Part print with two shaded views. Sizes in mm from the minimum x, y, z corner. A direction names the side the tool comes from. Coordinates: 2 decimals unless noted, no trailing zeros. Return JSON: item names as keys, results as strings. Group by question number.
(1) Flat gauge pins, fed straight in: pin 1 Ø12 at (x, z) = (252, 97) entering from -Y (3 decimals); pin 2 Ø3 at (x, y) = (267.5, 3.5) entering from +Z. Where does each tip first touch, or does it go through?
(2) Tool access for the marked faces 5 and 6: list every direction of +Z, -Z, +X, -X, +Y, -Y with a clear straight run to the whole face (end or side of a thin tool).
(3) Mould opens along Y. For the marked faces 1, 2, 3 and 4 say: pulls with the +Y half, pulls with the -Y half, needs draft (parallel to the pull), parting line crosses it, or undercut.
(4) Probe L1, parallel to Y at x = 463, z = 78 (1 decimal); L2, parallel to Z at x = 66.5, y = 49.5. List the from-to ranges inside material, lowest first.
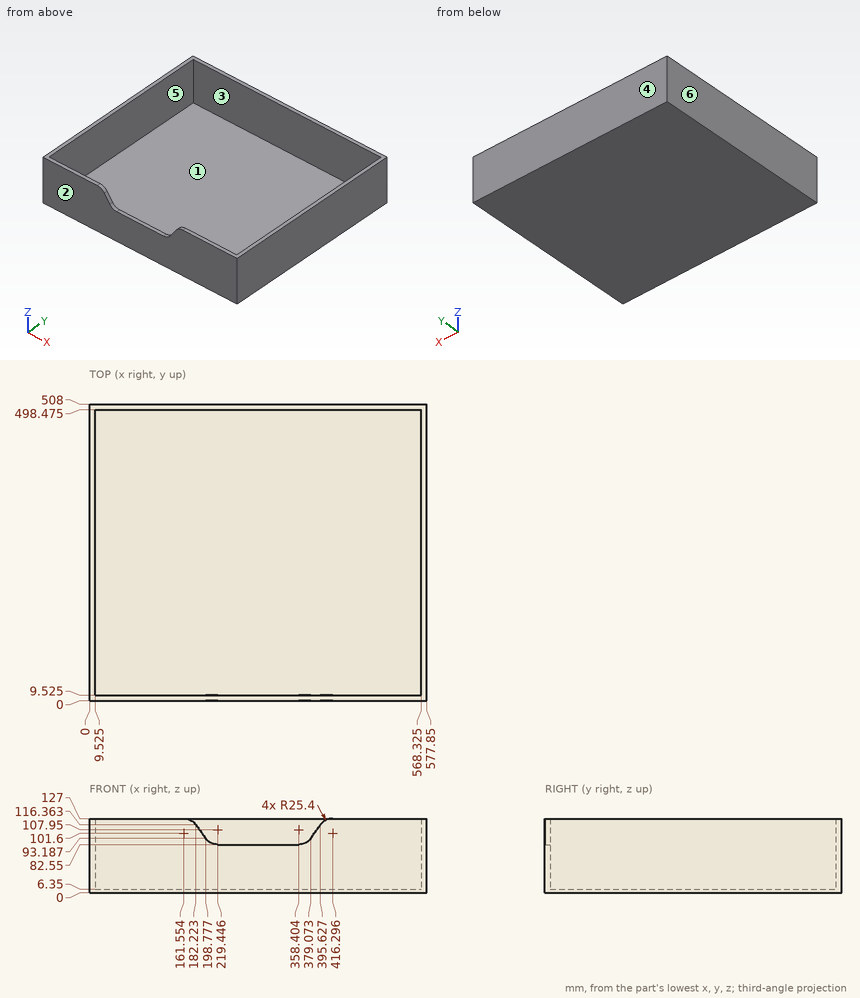
Geometry results:
{
 "1": {"pin 1": "y = 498.475", "pin 2": "z = 82.55"},
 "2": {"face 5": "+Z", "face 6": "+Z, -Z, -X, +Y, -Y"},
 "3": {"face 1": "undercut", "face 2": "pulls with the -Y half", "face 3": "undercut", "face 4": "pulls with the +Y half"},
 "4": {"L1": "0 to 9.5, 498.5 to 508", "L2": "0 to 6.35"}
}
